Verification items for the finished model (mm, model axes). A direction names the side the tool comes from. Coordinates: 2 decimals unless noted, no trailing zeros. Order: outer loops, then holes, each group sorted by start corner. A loop starts at its lowest first (then second) coordinate and runs counter-clockwise, first axis right, second up. Notation, with made-up numbers: (1.5, 11.25) -> (54.5, 11.25) arc R10 ccw to (54.5, 22.25) -> close; hole circle Ø10 at (73.25, 69). An arc over 180 degrees is marked (long way). Write item = value, one per line. Start each with the question number.
Autodesk Fusion 360 part; units mm, degrees
sketch "Sketch1" plane through (0, 0, 0) normal (0, 0, 1) x (1, 0, 0)
  line L0 (-15.25, 15.125) -> (15.25, 15.125)
  line L1 (15.25, 15.125) -> (15.25, -15.125)
  line L2 (15.25, -15.125) -> (-15.25, -15.125)
  line L3 (-15.25, -15.125) -> (-15.25, 15.125)
  line L4 (-15.25, 15.125) -> (15.25, -15.125) construction
  line L5 (15.25, 15.125) -> (-15.25, -15.125) construction
  dimension "d1" = 30.5
  dimension "d2" = 30.25
extrude "Extrude1" add sketch "Sketch1" along normal blind 1.6
sketch "Sketch2" plane through (0, 0, 1.6) normal (0, 0, 1) x (-1, 0, 0)
  line L0 (15.25, 15.125) -> (-15.25, 15.125)
  line L1 (-15.25, 15.125) -> (-15.25, -15.125)
  line L2 (-15.25, -15.125) -> (15.25, -15.125)
  line L3 (15.25, -15.125) -> (15.25, 15.125)
  line L4 (14, -15.125) -> (2, -15.125)
  line L5 (2, -15.125) -> (2, -4.125)
  line L6 (2, -4.125) -> (14, -4.125)
  line L7 (14, -4.125) -> (14, -15.125)
  line L8 (-2, -15.125) -> (-14, -15.125)
  line L9 (-14, -15.125) -> (-14, -4.125)
  line L10 (-14, -4.125) -> (-2, -4.125)
  line L11 (-2, -4.125) -> (-2, -15.125)
  dimension "d5" = 12
  dimension "d6" = 11
  dimension "d7" = 12
  dimension "d8" = 11
  dimension "d9" = 4
  dimension "d10" = 1.25
extrude "Extrude2" add sketch "Sketch2" along normal blind 5.5 contours L2 L4 L5 L6 L7 | L2 L8 L9 L10 L11
sketch "Sketch3" plane through (0, 15.125, 0) normal (0, 1, 0) x (-1, 0, 0)
  line L0 (-15.25, 0) -> (15.25, 0)
  line L1 (15.25, 0) -> (15.25, 1.6)
  line L2 (15.25, 1.6) -> (14, 1.6)
  line L3 (14, 1.6) -> (14, 7.1)
  line L4 (14, 7.1) -> (2, 7.1)
  line L5 (2, 7.1) -> (2, 1.6)
  line L6 (2, 1.6) -> (-2, 1.6)
  line L7 (-2, 1.6) -> (-2, 7.1)
  line L8 (-2, 7.1) -> (-14, 7.1)
  line L9 (-14, 7.1) -> (-14, 1.6)
  line L10 (-14, 1.6) -> (-15.25, 1.6)
  line L11 (-15.25, 1.6) -> (-15.25, 0)
  line L12 (-2, 1.6) -> (-14, 7.1) construction
  line L13 (2, 1.6) -> (14, 7.1) construction
  circle A0 centre (-8, 4.35) radius 3
  circle A1 centre (8, 4.35) radius 3
  circle A2 centre (-8, 4.35) radius 1.75
  circle A3 centre (8, 4.35) radius 1.75
  dimension "d13" = 6
  dimension "d14" = 6
  dimension "d15" = 3.5
  dimension "d16" = 3.5
extrude "Extrude3" add sketch "Sketch3" along normal blind 3 contours L8 A0 | L8 A0 | L4 A1 | L4 A1
chamfer "Chamfer1" distance 1.5 angle 45 4 edges at (-15.25, -15.125, 0.8) (-15.25, 15.125, 0.8) (15.25, -15.125, 0.8) (15.25, 15.125, 0.8)
sketch "Sketch4" plane through (0, 0, 0) normal (0, 0, -1) x (1, 0, 0)
  line L0 (13.75, -15.125) -> (15.25, -13.625)
  line L1 (15.25, -13.625) -> (15.25, 13.625)
  line L2 (15.25, 13.625) -> (13.75, 15.125)
  line L3 (13.75, 15.125) -> (-13.75, 15.125)
  line L4 (-13.75, 15.125) -> (-15.25, 13.625)
  line L5 (-15.25, 13.625) -> (-15.25, -13.625)
  line L6 (-15.25, -13.625) -> (-13.75, -15.125)
  line L7 (-13.75, -15.125) -> (13.75, -15.125)
  line L8 (0, -15.125) -> (0, 15.125) construction
  circle A0 centre (0, -12.25) radius 1.125
  circle A1 centre (12.625, 12.5) radius 1.125
  circle A2 centre (-12.625, 12.5) radius 1.125
  dimension "d20" = 2.25
  dimension "d21" = 1.75
  dimension "d22" = 1.5
  dimension "d23" = 1.5
  dimension "d24" = 1.5
  dimension "d25" = 1.5
  dimension "d26" = 2.25
  dimension "d27" = 2.25
extrude "Extrude4" cut sketch "Sketch4" against normal blind 1.6 contours A0 | A1 | A2
extrude "Extrude5" cut 2 faces at (7.9535, 15.125, 3.807) (-7.7869, 15.125, 4.893) along direction (0, -1, 0) blind 11
equation "d10 = ( 2.5 / 2 ) * 1 mm"
Item 1: Section check C-C (z = 0.75). Record the boundary of the cut face in (x, y) (3 decimals), then the cut area to 3 significant figures.
Item 2: Mould release check, pull along X, two halves, no side actions. Record for faces 6 (the flat face through (14, 10, 4)), 7 (the cylindrical face through (-8.941, 11.223, 5.826)), 8 (the cylindrical face through (5.14, 16.6, 3.45)), 9 (the flat face through (-8, 10, 7.1)): pulls with the +X half, pulls with the -X half, needs draft (parallel to the pull), parting line crosses it, or undercut.
Item 3: Section check D-D (z = 4.35). Record the boundary of the cut face in (x, y) (3 decimals).
Item 4: Tool access check on faces 1 (the flat face through (14.49, -14.386, 0.789)), 2 (the cylindrical face through (-10.86, 16.6, 3.45)), 3 (the cylindrical face through (-0.24, 13.35, 0.79)), 4 (the flat face through (9, 4.125, 6)), 5 (the flat face through (-2, 10, 4)). Record the directions out of +Z, -Z, +X, -X, +Y, -Y that give a thin tool (end or side, any length) a straight path to the whole face; none if there is none.
Item 5: Section check A-A (x = 0). Record the boundary of the cut face in (y, z) (3 decimals).
Item 6: Gauge pin test, flat ends, axial feed: P1, Ø12, axis at x = -5.5, y = -4, coming from the +Z side; P2, Ø1.6, axis at y = 12, z = 5.5, coming from the +X side; P3, Ø15, axis at x = 6.5, y = 4, coming from the +Z side. Record the tip position at first contact, or that the pin passes through.
Item 7: Section check B-B (y = 12.25). Record the boundary of the cut face in (x, z) (3 decimals), then the cut area to 3 significant figures.
Item 8: Thickness scan on line 1 (X direction, y = -12.5, z = 0.7); line 2 (X direction, y = 10.5, z = 2); line 3 (X direction, y = 12.25, z = 0.75) (3 decimals). Record the ranges inside material, lowest first.
Filled sheet:
q1.outline = (-15.25, -13.625) -> (-13.75, -15.125) -> (13.75, -15.125) -> (15.25, -13.625) -> (15.25, 13.625) -> (13.75, 15.125) -> (-13.75, 15.125) -> (-15.25, 13.625) -> close; hole circle Ø2.25 at (-12.625, -12.5); hole circle Ø2.25 at (0, 12.25); hole circle Ø2.25 at (12.625, -12.5)
q1.area = 906 mm^2
q2.face_6 = pulls with the +X half
q2.face_7 = undercut
q2.face_8 = undercut
q2.face_9 = needs draft
q3.outline = (-14, 4.125) -> (-9.75, 4.125) -> (-9.75, 18.125) -> (-11, 18.125) -> (-11, 15.125) -> (-13.75, 15.125) -> (-14, 14.875) -> close; (-6.25, 4.125) -> (-2, 4.125) -> (-2, 15.125) -> (-5, 15.125) -> (-5, 18.125) -> (-6.25, 18.125) -> close; (2, 4.125) -> (6.25, 4.125) -> (6.25, 18.125) -> (5, 18.125) -> (5, 15.125) -> (2, 15.125) -> close; (9.75, 4.125) -> (14, 4.125) -> (14, 14.875) -> (13.75, 15.125) -> (11, 15.125) -> (11, 18.125) -> (9.75, 18.125) -> close
q4.face_1 = +Z, -Z, +X, -Y
q4.face_2 = +Y
q4.face_3 = +Z, -Z
q4.face_4 = +Z, +X, -X, -Y
q4.face_5 = +Z, +Y, -Y
q5.outline = (-15.125, 0) -> (11.125, 0) -> (11.125, 1.6) -> (-15.125, 1.6) -> close; (13.375, 0) -> (15.125, 0) -> (15.125, 1.6) -> (13.375, 1.6) -> close
q6.P1 = 1.6
q6.P2 = 14
q6.P3 = 7.1
q7.outline = (-15.25, 0) -> (-1.125, 0) -> (-1.125, 1.6) -> (-2, 1.6) -> (-2, 7.1) -> (-14, 7.1) -> (-14, 1.6) -> (-15.25, 1.6) -> close; (1.125, 0) -> (15.25, 0) -> (15.25, 1.6) -> (14, 1.6) -> (14, 7.1) -> (2, 7.1) -> (2, 1.6) -> (1.125, 1.6) -> close; hole circle Ø3.5 at (-8, 4.35); hole circle Ø3.5 at (8, 4.35)
q7.area = 158 mm^2
q8.line_1 = -15.25 to -13.75, -11.5 to 11.5, 13.75 to 15.25
q8.line_2 = -14 to -2, 2 to 14
q8.line_3 = -15.25 to -1.125, 1.125 to 15.25
